from build123d import *

# Parameters (mm, degrees)
SKETCH4_W               = 100
SKETCH4_H               = 9
BOSS_EXTRUDE3_DEPTH     = 50
SKETCH5_R               = 42.5
CUT_EXTRUDE1_DEPTH      = 1
CUT_EXTRUDE1_DEPTH_BACK = 4


with BuildPart() as part:
    # Sketch4 → Boss-Extrude3 (new body, symmetric)
    with BuildSketch(Plane.YZ):
        with Locations((0, 4.5)):
            Rectangle(SKETCH4_W, SKETCH4_H)
    extrude(amount=BOSS_EXTRUDE3_DEPTH, both=True)

    # Sketch5 → Cut-Extrude1 (cut, two sides)
    with BuildSketch(Plane.XY.offset(9)) as cut_extrude1_sk:
        Circle(SKETCH5_R)
    extrude(amount=CUT_EXTRUDE1_DEPTH, mode=Mode.SUBTRACT)
    extrude(cut_extrude1_sk.sketch, amount=-CUT_EXTRUDE1_DEPTH_BACK, mode=Mode.SUBTRACT)


solid = part.part
Build history of the part. All positions in model axes, mm. A direction names the side the tool comes from. Give positions to 0.01 mm unless a question says otherwise; leave off trailing zeros. Loops run counter-clockwise (first coordinate to the right, second up) from the corner with the lowest first, then second, coordinate; pieces in that order, holes last. Notation, with made-up numbers: (62.25, -7.5) - (83.25, -7.5) arc R34 ccw to (83.25, 29.5) - close; hole circle Ø11 at (29.25, 8). An arc over 180 degrees is marked (long way). Write item = value, one per line. Start each with the question number.
1) Tool access for faces 1 (the flat face through (-50, -1, 5)), 2 (the flat face through (-1, 1, 5)): list every direction of +Z, -Z, +X, -X, +Y, -Y with a clear straight run to the whole face (end or side of a thin tool).
2) Drop a flat-ended pin along its axis: pin 1 Ø12 at (x, y) = (-28, -2.5) entering from -Z. Give the stop position or say it passes through.
3) Probe probe 1 along Y at (x, z) = (0, 7.3); probe 2 along Z at (x, y) = (-19, 32); probe 3 along X at (y, z) = (13, 8). List the from-to ranges inside material, lowest first. Write a range as from..to.
4) Band-saw the part on A-A on y = 0. Give the cut face in (x, z), plus the area to 3 significant figures.
5) Band-saw the part on B-B on x = -10. Give the cut face in (y, z), plus the area to 3 significant figures.
Final values:
q1.face_1 = +Z, -Z, -X, +Y, -Y
q1.face_2 = +Z
q2.pin_1 = 0
q3.probe_1 = -50..-42.5, 42.5..50
q3.probe_2 = 0..5
q3.probe_3 = -50..-40.46, 40.46..50
q4.outline = (-50, 0) - (50, 0) - (50, 9) - (42.5, 9) - (42.5, 5) - (-42.5, 5) - (-42.5, 9) - (-50, 9) - close
q4.area = 560 mm²
q5.outline = (-50, 0) - (50, 0) - (50, 9) - (41.31, 9) - (41.31, 5) - (-41.31, 5) - (-41.31, 9) - (-50, 9) - close
q5.area = 570 mm²
